Source: CAD feature listing. Evaluate the final solid. Frame: model axes, mm. A direction names the side the tool comes from. Give positions to 0.01 mm unless a question says otherwise; leave off trailing zeros. Order: outer loops, then holes, each group sorted by start corner. A loop starts at its lowest first (then second) coordinate and runs counter-clockwise, first axis right, second up. Notation, with made-up numbers: M 62.5,32 L 90.5,32 A25 ccw 90.5,66 Z; hole C -6.75,67 d6. An arc over 180 degrees is marked long. Answer as a JSON object with one key per item and string values. Group by question number.
1. Section query C-C (z = -202). Output: boundary loops of the cut face in (x, y).
2. Set-up query: faces 1 (the cylindrical face through (-14.9, 3.2, -52.7)), 2 (the flat face through (31.185, 3.131, -97.951)). Return all of +Z, -Z, +X, -X, +Y, -Y with unobstructed straight access to the full face (end or side cutting, diameter ignored); none if empty.
3. Section query B-B (z = -64). Output: boundary loops of the cut face in (x, y), plus the area to 3 significant figures.
4. Pull-direction query (X, two-part tool) for faces 3 (the flat face through (0, 0, -106)), 4 (the cylindrical face through (0.92, 3.22, -220.98)), 5 (the flat face through (-31.29, 3.13, -100.73)), 6 (the cylindrical face through (15.1, 3.2, -52.7)); classes: +X half, -X half, draft (parallel to the pull), parting line (faces both ways), or undercut.
5. Pin query (flat end, axial travel): P1, Ø1.5, axis at x = -10, y = 3, coming from the +Z side; P2, Ø3, axis at y = 3.5, z = -69.5, coming from the +X side; P3, Ø2.5, axis at x = -15.5, z = -148.5, coming from the +Y side; P4, Ø2, axis at x = 22.5, y = 2.5, coming from the +Z side. Return the tip coordinate at first contact, or that it passes through.
6. Material intervals for L1, parallel to Z at x = -0.5, y = 0.5; L2, parallel to X at y = 4.25, z = -117.5; L3, parallel to Z at x = 13.5, y = 2.75, sorted ascending. Write a range as [from, to].
7. Section query A-A (x = 8). Output: boundary loops of the cut face in (y, z), plus the area to 3 significant figures.
8. Section query D-D (y = 1.5). Count the separate pieces of the cut face and the enclosed holes in it, plus the area to 3 significant figures.
from build123d import *

# Parameters (mm, degrees)
BOSS_EXTRUDE1_DEPTH     = 6.35
SKETCH2_R               = 2.6
CUT_EXTRUDE1_DEPTH      = 238.676928834
ESQUISSE3_R             = 21
ENL_V_MAT_EXTRU_2_DEPTH = 238.676928834
ESQUISSE7_R             = 1.5
ENL_V_MAT_EXTRU_3_DEPTH = 238.676928834
CUT_EXTRUDE3_DEPTH      = 238.676928834
SKETCH5_R               = 1.5
CUT_EXTRUDE4_DEPTH      = 238.676928834


with BuildPart() as part:
    # Sketch1 → Boss-Extrude1 (new body)
    with BuildSketch(Plane(origin=(0, 0, 0), x_dir=(1, 0, 0), z_dir=(0, 1, 0))):
        with BuildLine():
            Line((27.5, 0), (34.975254116, 198.684097441))
            ThreePointArc((34.975254116, 198.684097441), (0, 235), (-34.975254116, 198.684097441))
            Line((-34.975254116, 198.684097441), (-27.5, 0))
            ThreePointArc((-27.5, 0), (0, -27.5), (27.5, 0))
        make_face()
    extrude(amount=BOSS_EXTRUDE1_DEPTH)

    # Sketch2 → Cut-Extrude1 (cut, through all)
    with BuildSketch(Plane(origin=(0, 6.35, 0), x_dir=(1, 0, 0), z_dir=(0, 1, 0))):
        with Locations(Location((0, 0, 0), (0, 0, 270))):
            Circle(SKETCH2_R)
    extrude(amount=-CUT_EXTRUDE1_DEPTH, mode=Mode.SUBTRACT)

    # Esquisse3 → Enlèv. mat.-Extru.2 (cut, through all)
    with BuildSketch(Plane(origin=(0, 6.35, 0), x_dir=(1, 0, 0), z_dir=(0, 1, 0))):
        with Locations(Location((0, 200, 0), (0, 0, 270))):
            Circle(ESQUISSE3_R)
    extrude(amount=-ENL_V_MAT_EXTRU_2_DEPTH, mode=Mode.SUBTRACT)

    # Esquisse7 → Enlèv. mat.-Extru.3 (cut, through all)
    with BuildSketch(Plane(origin=(0, 6.35, 0), x_dir=(1, 0, 0), z_dir=(0, 1, 0))):
        with Locations(Location((-19.339370465, 219.339370465, 0), (0, 0, 270))):
            Circle(ESQUISSE7_R)
        with Locations(Location((19.339370465, 219.339370465, 0), (0, 0, 270))):
            Circle(ESQUISSE7_R)
        with Locations(Location((19.339370465, 180.660629535, 0), (0, 0, 270))):
            Circle(ESQUISSE7_R)
        with Locations(Location((-19.339370465, 180.660629535, 0), (0, 0, 270))):
            Circle(ESQUISSE7_R)
    extrude(amount=-ENL_V_MAT_EXTRU_3_DEPTH, mode=Mode.SUBTRACT)

    # Sketch4 → Cut-Extrude3 (cut, through all)
    with BuildSketch(Plane(origin=(0, 6.35, 0), x_dir=(1, 0, 0), z_dir=(0, 1, 0))):
        with BuildLine():
            Line((-19, 56.7), (-19, 96.7))
            ThreePointArc((-19, 96.7), (-15, 100.7), (-11, 96.7))
            Line((-11, 96.7), (-11, 56.7))
            ThreePointArc((-11, 56.7), (-15, 52.7), (-19, 56.7))
        make_face()
        with BuildLine():
            Line((11, 56.7), (11, 96.7))
            ThreePointArc((11, 96.7), (15, 100.7), (19, 96.7))
            Line((19, 96.7), (19, 56.7))
            ThreePointArc((19, 56.7), (15, 52.7), (11, 56.7))
        make_face()
    extrude(amount=-CUT_EXTRUDE3_DEPTH, mode=Mode.SUBTRACT)

    # Sketch5 → Cut-Extrude4 (cut, through all)
    with BuildSketch(Plane.XZ):
        with Locations(Location((15.5, -117.5, 0), (0, 0, 270))):
            Circle(SKETCH5_R)
        with Locations(Location((15.5, -148.5, 0), (0, 0, 270))):
            Circle(SKETCH5_R)
        with Locations(Location((-15.5, -148.5, 0), (0, 0, 270))):
            Circle(SKETCH5_R)
        with Locations(Location((-15.5, -117.5, 0), (0, 0, 270))):
            Circle(SKETCH5_R)
    extrude(amount=-CUT_EXTRUDE4_DEPTH, mode=Mode.SUBTRACT)


solid = part.part
Answer sheet:
{
 "1": {"outline": "M -34.94,0 L -20.9,0 L -20.9,6.35 L -34.94,6.35 Z; M 20.9,0 L 34.94,0 L 34.94,6.35 L 20.9,6.35 Z"},
 "2": {"face 1": "+Y, -Y", "face 2": "+Z, +X, +Y, -Y"},
 "3": {"outline": "M -29.91,0 L -19,0 L -19,6.35 L -29.91,6.35 Z; M -11,0 L 11,0 L 11,6.35 L -11,6.35 Z; M 19,0 L 29.91,0 L 29.91,6.35 L 19,6.35 Z", "area": "278 mm^2"},
 "4": {"face 3": "draft", "face 4": "undercut", "face 5": "-X half", "face 6": "undercut"},
 "5": {"P1": "z = 25.9", "P2": "x = 30.17", "P3": "through", "P4": "z = 17.15"},
 "6": {"L1": "[-235, -220.99], [-179.01, -2.55], [2.55, 27.5]", "L2": "[-31.92, -17], [-14, 14], [17, 31.92]", "L3": "[-232.29, -216.09], [-183.91, -100.41], [-52.99, 23.96]"},
 "7": {"outline": "M 0,-234.07 L 6.35,-234.07 L 6.35,-219.42 L 0,-219.42 Z; M 0,-180.58 L 6.35,-180.58 L 6.35,26.31 L 0,26.31 Z", "area": "1,410 mm^2"},
 "8": {"separate pieces": "1", "enclosed holes": "12", "area": "13,400 mm^2"}
}
